```python
from build123d import *

# Parameters (mm, degrees)
F1_DEPTH = 571.5
F2_DEPTH = 25.4
F3_DEPTH = 571.5
F4_DEPTH = 25.4


with BuildPart() as f1:
    # F0 (on Top) → F1 (new body, symmetric)
    with BuildSketch(Plane.XY):
        Polygon((-50.8, 0), (0, 0), (0, 76.2), (-76.2, 76.2), (-76.2, 0), align=None)
    extrude(amount=F1_DEPTH, both=True)

    # F0 (on Top) → F2 (join)
    with BuildSketch(Plane.XY):
        Polygon((-177.8, 0), (-76.2, 0), (-76.2, 76.2), align=None)
        Polygon((0, 76.2), (0, 0), (101.6, 0), align=None)
    extrude(amount=F2_DEPTH)

    # F0 (on Top) → F3 (join, symmetric)
    with BuildSketch(Plane.XY):
        Polygon((-76.2, -228.6), (-76.2, 0), (-177.8, 0), (-203.2, 0), (-203.2, -228.6), align=None)
        Polygon((101.6, 0), (0, 0), (-50.8, 0), (-76.2, 0), (-76.2, -228.6), (101.6, -228.6), align=None)
    extrude(amount=F3_DEPTH, both=True)

    # F3_face (on face) → F4 (join)
    with BuildSketch(Plane(origin=(-49.823077, -102.576923, 571.5), x_dir=(1, 0, 0), z_dir=(0, 0, 1))):
        Polygon((-153.376923, 102.576923), (-153.376923, -126.023077), (151.423077, -126.023077), (151.423077, 102.576923), (49.823077, 102.576923), (49.823077, 178.776923), (-26.376923, 178.776923), (-26.376923, 102.576923), align=None)
    extrude(amount=F4_DEPTH)


solid = f1.part
```
Model file for the job. Use its own axes, mm. A direction names the side the tool comes from. Coordinates: 2 decimals unless noted, no trailing zeros. Order: outer loops, then holes, each group sorted by start corner. A loop starts at its lowest first (then second) coordinate and runs counter-clockwise, first axis right, second up. Notation, with made-up numbers: (27.5, 51) - (75.5, 51) arc R24 cw to (75.5, 70) - close; hole circle Ø4 at (-14.75, -2). An arc over 180 degrees is marked (long way). Return JSON: item names as keys, results as strings. Group by question number.
1) Saw through at A-A, the plane z = 163.5. Write the cut outline in (x, y).
2) Flat gauge pins, fed straight in: P1, Ø23, axis at x = -115, y = 42.5, coming from the +Z side; P2, Ø1, axis at y = 44, z = -339.5, coming from the +X side; P3, Ø23, axis at y = 57, z = 350.5, coming from the -X side. Where does each tip first touch, or does it go through?
3) Saw through at C-C, the plane z = 10. Write the cut outline in (x, y).
4) Tool access for faces 4 (the flat face through (-105, 22, 25.4)), 5 (the flat face through (0, 38, -282)), 6 (the flat face through (52, 0, 307)), 7 (the flat face through (-181, 0, 5)): list every direction of +Z, -Z, +X, -X, +Y, -Y with a clear straight run to the whole face (end or side of a thin tool).
5) Mould opens along Z. For faces 1 (the flat face through (-203.2, -113, 5)), 2 (the flat face through (-53, -108, 596.9)), 3 (the flat face through (-53, -108, -571.5)) say: released by +Z, released by -Z, zero draft, split by the parting line, or undercut.
6) Probe line 1 (Y direction, x = -104, z = 347); line 2 (Z direction, x = -88, y = 45); line 3 (X direction, y = 9, z = -78). List the from-to ranges inside material, lowest first. Write a range as from..to.
7) Saw through at D-D, the plane y = 20. Write the cut outline in (x, z).
8) Saw through at B-B, the plane x = -139. Write the cut outline in (y, z), plus the area to 3 significant figures.
Values found:
{
 "1": {"outline": "(-203.2, -228.6) - (101.6, -228.6) - (101.6, 0) - (0, 0) - (0, 76.2) - (-76.2, 76.2) - (-76.2, 0) - (-203.2, 0) - close"},
 "2": {"P1": "stops at z = 25.4", "P2": "stops at x = 0", "P3": "stops at x = -76.2"},
 "3": {"outline": "(-203.2, -228.6) - (101.6, -228.6) - (101.6, 0) - (0, 76.2) - (-76.2, 76.2) - (-177.8, 0) - (-203.2, 0) - close"},
 "4": {"face 4": "+Z, -X, +Y", "face 5": "-Z, +X, +Y", "face 6": "+Z, +X, +Y", "face 7": "-X, +Y"},
 "5": {"face 1": "zero draft", "face 2": "released by +Z", "face 3": "released by -Z"},
 "6": {"line 1": "y = -228.6..0", "line 2": "z = 0..25.4", "line 3": "x = -76.2..0"},
 "7": {"outline": "(-151.13, 0) - (-76.2, 0) - (-76.2, -571.5) - (0, -571.5) - (0, 0) - (74.93, 0) - (74.93, 25.4) - (0, 25.4) - (0, 596.9) - (-76.2, 596.9) - (-76.2, 25.4) - (-151.13, 25.4) - close"},
 "8": {"outline": "(-228.6, -571.5) - (0, -571.5) - (0, 0) - (29.1, 0) - (29.1, 25.4) - (0, 25.4) - (0, 596.9) - (-228.6, 596.9) - close", "area": "268,000 mm²"}
}
